Verification items for the finished model (mm, model axes). Face numbers are marked on the shaded views. A direction names the side the tool comes from. Coordinates: 2 decimals unless noted, no trailing zeros. Loops run counter-clockwise (first coordinate to the right, second up) from the corner with the lowest first, then second, coordinate; pieces in that order, holes last. Notation, with made-up numbers: (38, -7.75) - (57, -7.75) arc R19 ccw to (57, 27.25) - close; hole circle Ø10 at (60, 58). An arc over 180 degrees is marked (long way). One line per item, written item: value. Start each with the question number.
(1) Set-up check for the marked faces 1 and 2: record each of +Z, -Z, +X, -X, +Y, -Y from which the full face is reachable in a straight line by a thin tool's end or side.
(2) Draft check along Z on the marked faces 3, 4 and 5. Enter one of: +Z half, -Z half, draft (parallel to the pull), parting line (faces both ways), or undercut.
(3) Gauge pin test, flat ends, axial feed: P1, Ø12, axis at x = 22.5, y = -16, coming from the +Z side; P2, Ø11.5, axis at x = 11, z = 26, coming from the -Y side; P3, Ø5, axis at y = -22, z = 24.5, coming from the +X side; P4, Ø1, axis at y = -19, z = 5.5, coming from the +X side. Record the tip position at first contact, or that the pin passes through.
(4) Section check A-A (x = -10.5). Record the boundary of the cut face in (y, z).
(5) Section check B-B (z = 14). Record the boundary of the cut face in (x, y).
(6) Section check D-D (x = 10). Record the boundary of the cut face in (y, z), plus the area to 3 significant figures.
(7) Thickness scan on probe 1 along Z at (x, y) = (0, -6); probe 2 along Y at (x, z) = (15, 17); probe 3 along Z at (x, y) = (0, -18.75). Record the ranges inside material, lowest first. Write a range as [from, to].
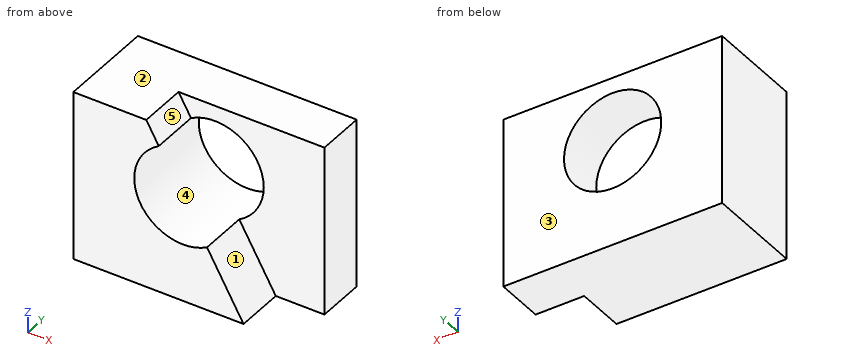
```python
from build123d import *

# Parameters (mm, degrees)
F0_W     = 57.15
F0_H     = 44.45
F1_DEPTH = 25.4
F3_DEPTH = 12.7
F4_R     = 12.7
F5_DEPTH = 27940


with BuildPart() as f1:
    # F0 (on Front) → F1 (new body)
    with BuildSketch(Plane.XZ):
        with Locations((-0.033397, 17.489623)):
            Rectangle(F0_W, F0_H)
    extrude(amount=F1_DEPTH)

    # F2 (on face) → F3 (cut)
    with BuildSketch(Plane.XZ.offset(25.4)):
        Polygon((28.541603, 39.714623), (-9.558397, 39.714623), (15.841603, -4.735377), (28.541603, -4.735377), align=None)
    extrude(amount=-F3_DEPTH, mode=Mode.SUBTRACT)

    # F4 (on face) → F5 (cut)
    with BuildSketch(Plane.XZ.offset(25.4)):
        with Locations((0, 22.987428)):
            Circle(F4_R)
    extrude(amount=-F5_DEPTH, mode=Mode.SUBTRACT)


solid = f1.part
```
Responses:
1. face 1: +Z, +X, -Y
1. face 2: +Z, +X, -X, +Y, -Y
2. face 3: draft
2. face 4: undercut
2. face 5: +Z half
3. P1: stops at z = 39.71
3. P2: stops at y = -12.7
3. P3: stops at x = -12.05
3. P4: stops at x = 10.28
4. outline: (-25.4, -4.74) - (0, -4.74) - (0, 15.84) - (-25.4, 15.84) - close; (-25.4, 30.13) - (0, 30.13) - (0, 39.71) - (-25.4, 39.71) - close
5. outline: (-28.61, -25.4) - (-8.97, -25.4) - (-8.97, 0) - (-28.61, 0) - close; (8.97, -12.7) - (28.54, -12.7) - (28.54, 0) - (8.97, 0) - close
6. outline: (-25.4, -4.74) - (0, -4.74) - (0, 15.16) - (-12.7, 15.16) - (-12.7, 5.49) - (-25.4, 5.49) - close; (-12.7, 30.82) - (0, 30.82) - (0, 39.71) - (-12.7, 39.71) - close
6. area: 495 mm²
7. probe 1: z = [-4.74, 10.29], [35.69, 39.71]
7. probe 2: y = [-12.7, 0]
7. probe 3: z = [-4.74, 10.29]
